Source: three-view drawing plus pictorial views. Frame: mm from the lowest corner of the part. A direction names the side the tool comes from. Round coordinates to 2 decimals unless told otherwise and drop trailing zeros. Loops run counter-clockwise (first coordinate to the right, second up) from the corner with the lowest first, then second, coordinate; pieces in that order, holes last. Notation, with made-up numbers: (19, 70.25) -> (60, 70.25) arc R19 cw to (60, 103.25) -> close; hole circle Ø4 at (33, 17). An arc over 180 degrees is marked (long way). Return JSON: item names as keys, results as strings. Group by question number.
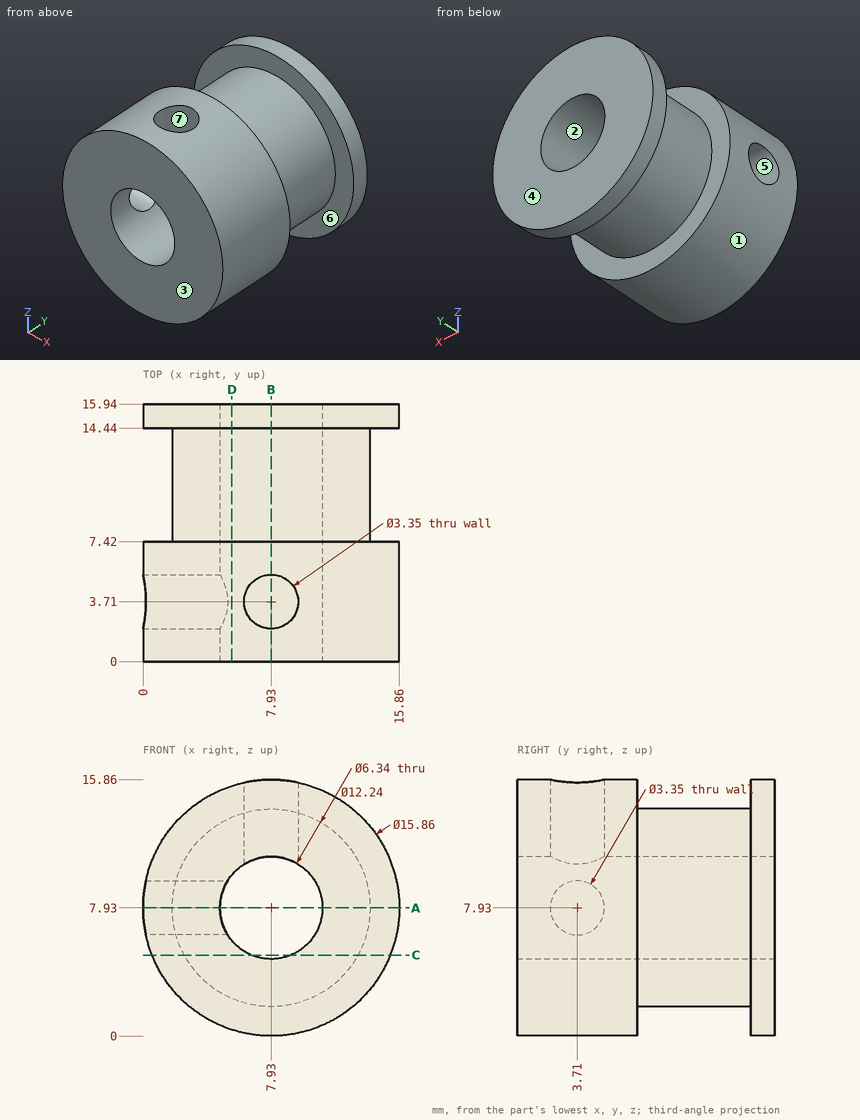
(1) Cut plane D-D (x = 5.5). Return loops of the section in (y, z).
(2) Mould query, pull axis Z, two halves, no side actions, for the marked faces 1, 2 and 3. Classes: released by +Z, released by -Z, zero draft, split by the parting line, or undercut.
(3) Cut plane C-C (z = 5). Return loops of the section in (x, y), and give its area (3 significant figures).
(4) Pin query (flat end, axial travel): pin 1 (4 mm diameter, centred on x = 10.5, y = 9, fed in from +Z); pin 2 (6 mm diameter, centred on x = 12, y = 12, fed in from +Z); pin 3 (4 mm diameter, centred on y = 9.5, z = 14, fed in from -X). Return the tip coordinate at first contact, or that it passes through.
(5) Cut plane A-A (z = 7.93). Return loops of the section in (x, y) (3 decimals), and give its area (3 significant figures).
(6) Cut plane B-B (x = 7.93). Return loops of the section in (y, z) (3 decimals).
(7) Set-up query: the marked faces 4, 5, 6 and 7. Return all of +Z, -Z, +X, -X, +Y, -Y with unobstructed straight access to the full face (end or side cutting, diameter ignored); none if empty.
(8) Ray query, line 1 (Y direction, x = 8, z = 14.5); line 2 (Z direction, x = 7.93, y = 12.25); line 3 (Y direction, x = 1.75, z = 7). Return the intervals inside material, ascending.
Answers follow:
{
 "1": {"outline": "(0, 0.38) -> (7.42, 0.38) -> (7.42, 2.31) -> (14.44, 2.31) -> (14.44, 0.38) -> (15.94, 0.38) -> (15.94, 5.89) -> (0, 5.89) -> close; (0, 9.97) -> (15.94, 9.97) -> (15.94, 15.48) -> (14.44, 15.48) -> (14.44, 13.55) -> (7.42, 13.55) -> (7.42, 15.48) -> (0, 15.48) -> close"},
 "2": {"face 1": "split by the parting line", "face 2": "undercut", "face 3": "zero draft"},
 "3": {"outline": "(0.56, 0) -> (6.72, 0) -> (6.72, 15.94) -> (0.56, 15.94) -> (0.56, 14.44) -> (2.56, 14.44) -> (2.56, 7.42) -> (0.56, 7.42) -> close; (9.14, 0) -> (15.3, 0) -> (15.3, 7.42) -> (13.3, 7.42) -> (13.3, 14.44) -> (15.3, 14.44) -> (15.3, 15.94) -> (9.14, 15.94) -> close", "area": "168 mm^2"},
 "4": {"pin 1": "z = 15.75", "pin 2": "z = 15.51", "pin 3": "x = 3.36"},
 "5": {"outline": "(0, 0) -> (4.76, 0) -> (4.76, 2.035) -> (0, 2.035) -> close; (0, 5.385) -> (4.76, 5.385) -> (4.76, 15.94) -> (0, 15.94) -> (0, 14.44) -> (1.81, 14.44) -> (1.81, 7.42) -> (0, 7.42) -> close; (11.1, 0) -> (15.86, 0) -> (15.86, 7.42) -> (14.05, 7.42) -> (14.05, 14.44) -> (15.86, 14.44) -> (15.86, 15.94) -> (11.1, 15.94) -> close", "area": "110 mm^2"},
 "6": {"outline": "(0, 0) -> (7.42, 0) -> (7.42, 1.81) -> (14.44, 1.81) -> (14.44, 0) -> (15.94, 0) -> (15.94, 4.76) -> (0, 4.76) -> close; (0, 11.1) -> (2.035, 11.1) -> (2.035, 15.86) -> (0, 15.86) -> close; (5.385, 11.1) -> (15.94, 11.1) -> (15.94, 15.86) -> (14.44, 15.86) -> (14.44, 14.05) -> (7.42, 14.05) -> (7.42, 15.86) -> (5.385, 15.86) -> close"},
 "7": {"face 4": "+Z, -Z, +X, -X, +Y", "face 5": "-X", "face 6": "none", "face 7": "+Z"},
 "8": {"line 1": "0 to 2.04, 5.38 to 7.42, 14.44 to 15.94", "line 2": "1.81 to 4.76, 11.1 to 14.05", "line 3": "0 to 2.32, 5.1 to 7.42, 14.44 to 15.94"}
}
